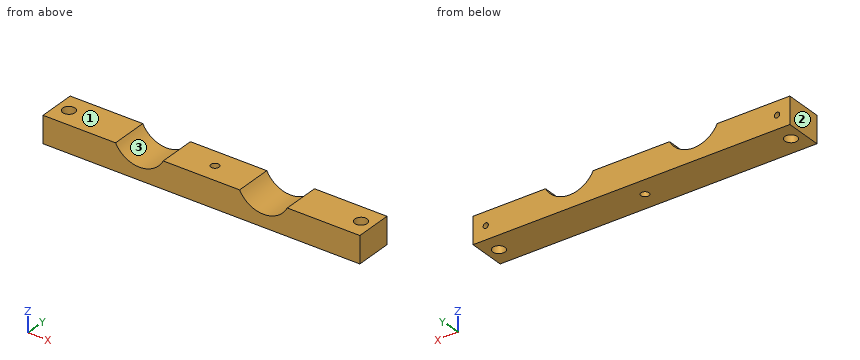
from build123d import *

# Parameters (mm, degrees)
BOSS_EXTRUDE1_DEPTH         = 19.05
F_1_4_0_25_DIAMETER_HOLE1_D = 6.35
F_6_32_TAPPED_HOLE1_REACH   = 86.612
F_6_32_TAPPED_HOLE1_BORE_R  = 1.35255
F_10_32_TAPPED_HOLE1_D      = 4.0386


with BuildPart() as part:
    # Sketch1 → Boss-Extrude1 (new body)
    with BuildSketch(Plane(origin=(0, 0, 0), x_dir=(1, 0, 0), z_dir=(0, 1, 0))):
        with BuildLine():
            Line((-19.59069957, 0), (19.59069957, 0))
            ThreePointArc((19.59069957, 0), (31.81985, 7.4295), (44.04900043, 0))
            Line((44.04900043, 0), (81.28, 0))
            Line((81.28, 0), (81.28, 13.7795))
            Line((81.28, 13.7795), (-81.28, 13.7795))
            Line((-81.28, 13.7795), (-81.28, 0))
            Line((-81.28, 0), (-44.04900043, 0))
            ThreePointArc((-44.04900043, 0), (-31.81985, 7.4295), (-19.59069957, 0))
        make_face()
    extrude(amount=BOSS_EXTRUDE1_DEPTH)

    # 1/4 (0.25) Diameter Hole1 (through all)
    with Locations(Plane.XY):
        with Locations((-74.93, 9.525)):
            f_1_4_0_25_diameter_hole1 = Hole(F_1_4_0_25_DIAMETER_HOLE1_D / 2)

    # #6-32 Tapped Hole1 bore → #6-32 Tapped Hole1 (cut, up to next)
    with BuildSketch(Plane(origin=(0, 19.05, 0), x_dir=(1, 0, 0), z_dir=(0, 1, 0)), mode=Mode.PRIVATE) as f_6_32_tapped_hole1_sk1:
        with Locations((-74.72934, 6.88975)):
            Circle(F_6_32_TAPPED_HOLE1_BORE_R)
    f_6_32_tapped_hole1_tool1 = extrude(f_6_32_tapped_hole1_sk1.sketch, amount=-F_6_32_TAPPED_HOLE1_REACH, mode=Mode.PRIVATE) & part.part
    f_6_32_tapped_hole1 = f_6_32_tapped_hole1_tool1.solids().sort_by_distance((-74.72934, 19.05, -6.88975))[0]
    add(f_6_32_tapped_hole1, mode=Mode.SUBTRACT)

    # Mirror2: 1/4 (0.25) Diameter Hole1, #6-32 Tapped Hole1 across plane
    add(f_1_4_0_25_diameter_hole1.mirror(Plane(origin=(0, 0, 0), x_dir=(0, 0, 1), z_dir=(1, 0, 0))), mode=Mode.SUBTRACT)
    add(f_6_32_tapped_hole1.mirror(Plane(origin=(0, 0, 0), x_dir=(0, 0, 1), z_dir=(1, 0, 0))), mode=Mode.SUBTRACT)

    # #10-32 Tapped Hole1 (through all)
    with Locations(Plane.XY):
        with Locations((0, 9.525)):
            Hole(F_10_32_TAPPED_HOLE1_D / 2)


solid = part.part
Verification items for the finished model (mm, model axes). Face numbers are marked on the shaded views. Coordinates: 2 decimals unless noted, no trailing zeros. Order: outer loops, then holes, each group sorted by start corner. A loop starts at its lowest first (then second) coordinate and runs counter-clockwise, first axis right, second up. Notation, with made-up numbers: M -36.75,7.25 L 22.25,7.25 A25 cw 22.25,36.25 Z; hole C 29,-39 d10. An arc over 180 degrees is marked long. Return JSON: item names as keys, results as strings.
1) Cross-section at C-C, the plane y = 4. Record the boundary of the cut face in (x, z), and give its area (3 significant figures).
Answer list:
{"outline": "M -81.28,-13.78 L 81.28,-13.78 L 81.28,0 L 44.05,0 A13.78 cw 19.59,0 L -19.59,0 A13.78 cw -44.05,0 L -81.28,0 Z", "area": "1,980 mm2"}
2) Cross-section at B-B, the plane z = -1.75. Record the boundary of the cut face in (x, y) (3 decimals).
Answer list:
{"outline": "M -81.28,0 L -42.967,0 L -42.967,19.05 L -81.28,19.05 Z; M -20.672,0 L 20.672,0 L 20.672,19.05 L -20.672,19.05 Z; M 42.967,0 L 81.28,0 L 81.28,19.05 L 42.967,19.05 Z; hole C -74.93,9.525 d6.35; hole C 0,9.525 d4.039; hole C 74.93,9.525 d6.35"}
3) Release check for a two-part mould opening along X. For the marked faces 1, 2 and 3 record: +X half, -X half, draft (parallel to the pull), parting line (faces both ways), or undercut.
Answer list:
{"face 1": "draft", "face 2": "-X half", "face 3": "undercut"}
4) Thickness scan on L1, parallel to X at y = 15.5, z = -6.25; L2, parallel to X at y = 10.5, z = -2; L3, parallel to X at y = 1, z = -2.25. Record the ranges inside material, lowest first. Write a range as [from, to].
Answer list:
{"L1": "[-81.28, -75.92], [-73.54, -37.4], [-26.24, 26.24], [37.4, 73.54], [75.92, 81.28]", "L2": "[-81.28, -77.95], [-71.91, -42.78], [-20.86, -1.77], [1.77, 20.86], [42.78, 71.91], [77.95, 81.28]", "L3": "[-81.28, -42.59], [-21.05, 21.05], [42.59, 81.28]"}
5) Cross-section at D-D, the plane z = -11.25. Record the boundary of the cut face in (x, y) (3 decimals).
Answer list:
{"outline": "M -81.28,0 L 81.28,0 L 81.28,19.05 L -81.28,19.05 Z; hole C -74.93,9.525 d6.35; hole C 0,9.525 d4.039; hole C 74.93,9.525 d6.35"}
6) Gauge pin test, flat end, axial feed: pin 1 (5 mm diameter, centred on x = 74.93, y = 9.525, fed in from +Z). Record the tip position at first contact, or that the pin passes through.
Answer list:
{"pin 1": "through"}
7) Cross-section at A-A, the plane x = 0. Record the boundary of the cut face in (y, z).
Answer list:
{"outline": "M 0,-13.78 L 7.51,-13.78 L 7.51,0 L 0,0 Z; M 11.54,-13.78 L 19.05,-13.78 L 19.05,0 L 11.54,0 Z"}
